Geometry check sheet. Reference: the model listing, model coordinates, mm. Round coordinates to 2 decimals unless told otherwise and drop trailing zeros. Write each loop counter-clockwise with the first axis right and the second up, starting at its lowest first coordinate (ties: lowest second). Pieces come first, ordered by that corner, then holes. Notation, with made-up numbers: M 47.5,-3.75 L 98.5,-3.75 A22 ccw 98.5,17.25 Z; hole C 71.25,-10.5 d3. An arc over 180 degrees is marked long. Put each result on its own line as item: value. Start each with the question number.
(1) Material ranges on probe 1 along X at (y, z) = (1.85, -1); probe 2 along X at (y, z) = (1.15, -0.5); probe 3 along Z at (x, y) = (98.5, 1.15), recorded low to high.
(2) Section check A-A on z = 0. Record the cut outline in (x, y).
(3) Mould release check, pull along Z, two halves, no side actions. Record for faces 1 (the flat face through (-2, 0, 0)), 2 (the cylindrical face through (-98.11, 0.99, 1.52)): pulls with the +Z half, pulls with the -Z half, needs draft (parallel to the pull), parting line crosses it, or undercut.
from build123d import *

# Parameters (mm, degrees)
SKETCH1_W                 = 220.18723
SKETCH1_H                 = 12
BOSS_EXTRUDE1_DEPTH       = 2
F_5_0MM_DOWEL_HOLE1_D     = 5
F_5_0MM_DOWEL_HOLE1_DEPTH = 2


with BuildPart() as part:
    # Sketch1 → Boss-Extrude1 (new body)
    with BuildSketch(Plane(origin=(0, 0, 0), x_dir=(1, 0, 0), z_dir=(0, 1, 0))):
        Rectangle(SKETCH1_W, SKETCH1_H)
    extrude(amount=BOSS_EXTRUDE1_DEPTH)

    # Ø5.0mm Dowel Hole1
    with Locations(Plane(origin=(0, 2, 0), x_dir=(1, 0, 0), z_dir=(0, 1, 0))):
        with Locations((-100.093615, 0), (100.093615, 0)):
            Hole(F_5_0MM_DOWEL_HOLE1_D / 2, depth=F_5_0MM_DOWEL_HOLE1_DEPTH)


solid = part.part
Answers follow:
1. probe 1: x = -110.09 to -102.38, -97.8 to 97.8, 102.38 to 110.09
1. probe 2: x = -110.09 to -102.54, -97.64 to 97.64, 102.54 to 110.09
1. probe 3: z = -6 to -1.93, 1.93 to 6
2. outline: M -110.09,0 L -102.59,0 L -102.59,2 L -110.09,2 Z; M -97.59,0 L 97.59,0 L 97.59,2 L -97.59,2 Z; M 102.59,0 L 110.09,0 L 110.09,2 L 102.59,2 Z
3. face 1: needs draft
3. face 2: undercut
